Verification items for the finished model (mm, model axes). Face numbers are marked on the shaded views. Coordinates: 2 decimals unless noted, no trailing zeros. Write each loop counter-clockwise with the first axis right and the second up, starting at its lowest first coordinate (ties: lowest second). Pieces come first, ordered by that corner, then holes. Notation, with made-up numbers: (-5.5, -22) -> (11.5, -22) arc R20 ccw to (11.5, 16) -> close; hole circle Ø8 at (45, 23). An arc over 180 degrees is marked (long way). Write item = value, one per line. Start each with the question number.
(1) Section check A-A (z = -10.5). Record the cut outline in (x, y) (3 decimals), plus the area to 3 significant figures.
(2) Material ranges on probe 1 along Y at (x, z) = (0, 3.95) (3 decimals); probe 2 along Y at (x, z) = (0, 6.3) (3 decimals); probe 3 along Z at (x, y) = (-63, 42), recorded low to high. Write a range as [from, to].
(3) Mould release check, pull along Y, two halves, no side actions. Record for the marked faces 1, 2 and 3: released by +Y, released by -Y, zero draft, split by the parting line, or undercut.
(4) Gauge pin test, flat ends, axial feed: pin 1 Ø16.5 at (y, z) = (-10.5, -8) entering from +X; pin 2 Ø21.5 at (x, y) = (0, 0) entering from -Z; pin 3 Ø12 at (x, z) = (35, -2) entering from +Y; pin 4 Ø1 at (x, y) = (26.5, 29.5) entering from -Z. Record the tip position at first contact, or that the pin passes through.
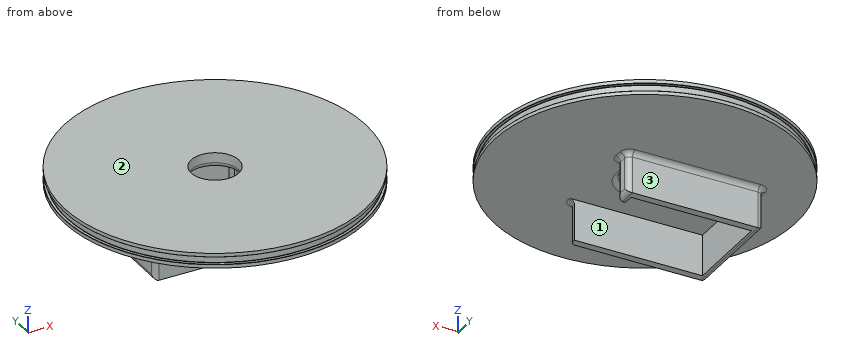
```python
from build123d import *
from OCP.BRepFilletAPI import BRepFilletAPI_MakeChamfer

# Parameters (mm, degrees)
SKETCH1_R           = 76.2
BOSS_EXTRUDE1_DEPTH = 7.62
CHAMFER1_SIZE       = 0.13
CHAMFER1_SIZE2      = 0.143008173
SKETCH3_R           = 12.065
CUT_EXTRUDE1_DEPTH  = 7.62
SKETCH4_W           = 68.58
SKETCH4_H           = 52.580948596
SKETCH4_W_2         = 60.96
SKETCH4_H_2         = 44.960948596
BOSS_EXTRUDE2_DEPTH = 20.828
SKETCH5_W           = 3.81
SKETCH5_H           = 39.880948596
CUT_EXTRUDE3_DEPTH  = 20.828
FILLET1_R           = 2.54


with BuildPart() as part:
    # Sketch1 → Boss-Extrude1 (new body)
    with BuildSketch(Plane.XY):
        with Locations(Location((0, 0, 0), (0, 0, 180))):
            Circle(SKETCH1_R)
    extrude(amount=BOSS_EXTRUDE1_DEPTH)

    # Sketch2 → Cut-Revolve1 (revolve, cut)
    with BuildSketch(Plane(origin=(0, 0, 0), x_dir=(0, 0, -1), z_dir=(1, 0, 0)), mode=Mode.PRIVATE) as cut_revolve1_sk:
        Polygon((-1.907556125, 76.2), (-2.032, 74.7776), (-5.588, 74.7776), (-5.712443875, 76.2), align=None)
    revolve(cut_revolve1_sk.sketch.rotate(Axis((0, 0, 0), (0, 0, 1)), 90), axis=Axis((0, 0, 0), (0, 0, 1)), mode=Mode.SUBTRACT)

    # Chamfer1: one chamfer whose edges measure the first distance from different faces: ONE call of the kernel's chamfer builder (chamfer() names one face for all edges)
    chamfer1_edges_1 = [part.edges().sort_by_distance(p)[0] for p in [
        (76.2, 0, 5.712443875),
    ]]
    chamfer1_side_1 = [part.faces().sort_by_distance(p)[0] for p in [
        (76.2, 0, 6.666221937),
    ]]
    chamfer1_edges_2 = [part.edges().sort_by_distance(p)[0] for p in [
        (76.2, 0, 1.907556125),
    ]]
    chamfer1_side_2 = [part.faces().sort_by_distance(p)[0] for p in [
        (75.4888, 0, 1.969778063),
    ]]
    chamfer1_edges_3 = [part.edges().sort_by_distance(p)[0] for p in [
        (74.7776, 0, 2.032),
    ]]
    chamfer1_side_3 = [part.faces().sort_by_distance(p)[0] for p in [
        (74.7776, 0, 3.81),
    ]]
    chamfer1_edges_4 = [part.edges().sort_by_distance(p)[0] for p in [
        (74.7776, 0, 5.588),
    ]]
    chamfer1_side_4 = [part.faces().sort_by_distance(p)[0] for p in [
        (75.4888, 0, 5.650221937),
    ]]
    chamfer1 = BRepFilletAPI_MakeChamfer(part.part.solid().wrapped)
    for e in chamfer1_edges_1:
        chamfer1.Add(CHAMFER1_SIZE, CHAMFER1_SIZE2, e.wrapped, chamfer1_side_1[0].wrapped)  # the first distance lies on this face
    for e in chamfer1_edges_2:
        chamfer1.Add(CHAMFER1_SIZE, CHAMFER1_SIZE2, e.wrapped, chamfer1_side_2[0].wrapped)  # the first distance lies on this face
    for e in chamfer1_edges_3:
        chamfer1.Add(CHAMFER1_SIZE, CHAMFER1_SIZE2, e.wrapped, chamfer1_side_3[0].wrapped)  # the first distance lies on this face
    for e in chamfer1_edges_4:
        chamfer1.Add(CHAMFER1_SIZE, CHAMFER1_SIZE2, e.wrapped, chamfer1_side_4[0].wrapped)  # the first distance lies on this face
    add(Compound.cast(chamfer1.Shape()), mode=Mode.REPLACE)

    # Sketch3 → Cut-Extrude1 (cut)
    with BuildSketch(Plane.XY.offset(7.62)):
        Circle(SKETCH3_R)
    extrude(amount=-CUT_EXTRUDE1_DEPTH, mode=Mode.SUBTRACT)

    # Sketch4 → Boss-Extrude2 (add)
    with BuildSketch(Plane(origin=(0, 0, 0), x_dir=(-1, 0, 0), z_dir=(0, 0, -1))):
        with Locations((14.605, -6.605474298)):
            Rectangle(SKETCH4_W, SKETCH4_H)
        with Locations((14.605, -6.605474298)):
            Rectangle(SKETCH4_W_2, SKETCH4_H_2, mode=Mode.SUBTRACT)
    extrude(amount=BOSS_EXTRUDE2_DEPTH)

    # Sketch5 → Cut-Extrude3 (cut)
    with BuildSketch(Plane(origin=(0, 0, -20.828), x_dir=(-1, 0, 0), z_dir=(0, 0, -1))):
        with Locations((-17.78, -9.145474298)):
            Rectangle(SKETCH5_W, SKETCH5_H)
    extrude(amount=-CUT_EXTRUDE3_DEPTH, mode=Mode.SUBTRACT)

    # Fillet1
    fillet1_edges = [part.edges().sort_by_distance(p)[0] for p in [
        (-12.065, 0, 0),
        (19.685, -30.990948596, 0),
        (17.78, 10.795, 0),
        (-14.605, -32.895948596, 0),
        (-14.605, 19.685, 0),
        (19.685, 19.685, -10.414),
        (19.685, 15.24, -20.828),
        (19.685, 10.795, -10.414),
        (19.685, 15.24, 0),
        (-48.895, -32.895948596, -10.414),
        (-48.895, -6.605474298, -20.828),
        (-48.895, 19.685, -10.414),
        (-48.895, -6.605474298, 0),
        (19.685, -32.895948596, -10.414),
    ]]
    fillet(fillet1_edges, radius=FILLET1_R)


solid = part.part
```
Response:
q1.outline = (-48.895, -30.356) arc R2.54 ccw to (-46.355, -32.896) -> (17.145, -32.896) arc R2.54 ccw to (19.685, -30.356) -> (19.685, -29.086) -> (-45.085, -29.086) -> (-45.085, 15.875) -> (15.875, 15.875) -> (15.875, 10.795) -> (17.145, 10.795) arc R2.54 ccw to (19.685, 13.335) -> (19.685, 17.145) arc R2.54 ccw to (17.145, 19.685) -> (-46.355, 19.685) arc R2.54 ccw to (-48.895, 17.145) -> close
q1.area = 706 mm2
q2.probe_1 = [-74.778, -12.065], [12.065, 74.778]
q2.probe_2 = [-76.2, -12.065], [12.065, 76.2]
q2.probe_3 = [0, 1.95], [5.67, 7.62]
q3.face_1 = undercut
q3.face_2 = zero draft
q3.face_3 = released by +Y
q4.pin_1 = 75.73
q4.pin_2 = through
q4.pin_3 = 70.32
q4.pin_4 = 0
